Could you check a few things on this model? Use its own coordinates, in mm. Coordinates: 2 decimals unless noted, no trailing zeros. Loops run counter-clockwise (first coordinate to the right, second up) from the corner with the lowest first, then second, coordinate; pieces in that order, holes last. Notation, with made-up numbers: M -34.75,43.25 L -5.75,43.25 A16 ccw -5.75,65.25 Z; hole C -12.5,-18 d5. An arc over 180 degrees is marked long. Use one line per item in the form item = value. Start each with the question number.
Autodesk Inventor part; units mm, degrees
ref_plane "YZ Plane" through (0, 0, 0) normal (1, 0, 0) x (0, 1, 0)
ref_plane "XZ Plane" through (0, 0, 0) normal (0, 1, 0) x (-1, 0, 0)
ref_plane "XY Plane" through (0, 0, 0) normal (0, 0, 1) x (1, 0, 0)
sketch "Sketch1" plane through (0, 0, 0) normal (0, 1, 0) x (-1, 0, 0)
  line L0 (-100.9651, 48.6333) -> (-100.9651, -1.3667)
  line L1 (79.933, 58.6333) -> (-90.9651, 58.6333)
  line L2 (145.3335, 17.5604) -> (88.3289, 56.0635)
  line L3 (-100.9651, -1.3667) -> (-100.9651, -51.3667)
  circle A0 centre (115.0349, 25.6333) radius 1.6
  circle A1 centre (115.0349, -28.3667) radius 1.6
  circle A2 centre (142.5349, 7.3833) radius 1.6
  circle A3 centre (142.5349, -10.1167) radius 1.6
  circle A4 centre (-94.3651, -9.7667) radius 1.6
  circle A5 centre (-94.3651, 7.0333) radius 1.6
  line L4 (147.5349, -16.1504) -> (147.5349, 13.417)
  arc A6 (-100.9651, -51.3667) -> (-90.9651, -61.3667) centre (-90.9651, -51.3667) ccw
  arc A7 (-90.9651, 58.6333) -> (-100.9651, 48.6333) centre (-90.9651, 48.6333) ccw
  arc A8 (88.3289, 56.0635) -> (79.933, 58.6333) centre (79.933, 43.6333) ccw
  arc A9 (79.933, -61.3667) -> (88.3289, -58.7969) centre (79.933, -46.3667) ccw
  arc A10 (147.5349, 13.417) -> (145.3335, 17.5604) centre (142.5349, 13.417) ccw
  arc A11 (145.3335, -20.2938) -> (147.5349, -16.1504) centre (142.5349, -16.1504) ccw
  line L5 (-90.9651, -61.3667) -> (79.933, -61.3667)
  line L6 (88.3289, -58.7969) -> (145.3335, -20.2938)
  line L7 (-90.9651, -1.3667) -> (-90.9651, 16.6333)
  line L8 (-89.9651, 17.6333) -> (-73.9651, 17.6333)
  arc A12 (-71.9651, 15.6333) -> (-73.9651, 17.6333) centre (-73.9651, 15.6333) ccw
  arc A13 (-89.9651, 17.6333) -> (-90.9651, 16.6333) centre (-89.9651, 16.6333) ccw
  line L9 (-71.9651, 15.6333) -> (-71.9651, -13.3667)
  line L10 (-83.9651, -20.3667) -> (-89.9651, -20.3667)
  arc A14 (-90.9651, -19.3667) -> (-89.9651, -20.3667) centre (-89.9651, -19.3667) ccw
  line L11 (-90.9651, -19.3667) -> (-90.9651, -1.3667)
  line L12 (16.0349, -17.3667) -> (16.0349, -43.3667)
  arc A15 (14.0349, -45.3667) -> (16.0349, -43.3667) centre (14.0349, -43.3667) ccw
  line L13 (14.0349, -15.3667) -> (-69.9651, -15.3667)
  arc A16 (16.0349, -17.3667) -> (14.0349, -15.3667) centre (14.0349, -17.3667) ccw
  arc A17 (-71.9651, -13.3667) -> (-69.9651, -15.3667) centre (-69.9651, -13.3667) ccw
  line L14 (14.0349, -45.3667) -> (-79.9651, -45.3667)
  arc A18 (-81.9651, -43.3667) -> (-79.9651, -45.3667) centre (-79.9651, -43.3667) ccw
  line L15 (-81.9651, -43.3667) -> (-81.9651, -22.3667)
  arc A19 (-81.9651, -22.3667) -> (-83.9651, -20.3667) centre (-83.9651, -22.3667) ccw
  line L16 (-54.6151, -49.4667) -> (-64.3151, -49.4667)
  line L17 (-64.3151, -49.4667) -> (-64.3151, -52.2667)
  line L18 (-59.4651, -52.2667) -> (-54.6151, -52.2667)
  line L19 (-54.6151, -52.2667) -> (-54.6151, -49.4667)
  line L20 (-59.4651, -52.2667) -> (-64.3151, -52.2667)
  line L21 (-79.6151, -49.4667) -> (-89.3151, -49.4667)
  line L22 (-89.3151, -49.4667) -> (-89.3151, -52.2667)
  line L23 (-84.4651, -52.2667) -> (-79.6151, -52.2667)
  line L24 (-79.6151, -52.2667) -> (-79.6151, -49.4667)
  line L25 (-84.4651, -52.2667) -> (-89.3151, -52.2667)
  line L26 (-54.6151, 46.7333) -> (-64.3151, 46.7333)
  line L27 (-64.3151, 46.7333) -> (-64.3151, 49.5333)
  line L28 (-59.4651, 49.5333) -> (-54.6151, 49.5333)
  line L29 (-54.6151, 49.5333) -> (-54.6151, 46.7333)
  line L30 (-59.4651, 49.5333) -> (-64.3151, 49.5333)
  line L31 (-79.6151, 46.7333) -> (-89.3151, 46.7333)
  line L32 (-89.3151, 46.7333) -> (-89.3151, 49.5333)
  line L33 (-84.4651, 49.5333) -> (-79.6151, 49.5333)
  line L34 (-79.6151, 49.5333) -> (-79.6151, 46.7333)
  line L35 (-84.4651, 49.5333) -> (-89.3151, 49.5333)
  circle A20 centre (-45.4651, -11.3667) radius 1.6
  circle A21 centre (-45.4651, 40.6333) radius 1.6
  circle A22 centre (86.5349, 40.6333) radius 1.6
  circle A23 centre (20.0349, -41.3667) radius 1.6
  circle A24 centre (86.5349, -41.3667) radius 1.6
  line L36 (129.6349, -6.5167) -> (129.6349, -24.2167)
  line L37 (132.4349, -6.5167) -> (132.4349, -24.2167)
  line L38 (129.6349, 3.7833) -> (129.6349, 21.4833)
  line L39 (132.4349, 3.7833) -> (132.4349, 21.4833)
  line L40 (119.3849, -2.7667) -> (94.6849, -2.7667)
  line L41 (94.6849, 0.0333) -> (119.3849, 0.0333)
  line L42 (94.6849, 0.0333) -> (94.6849, -2.7667)
  line L43 (119.3849, 0.0333) -> (119.3849, -2.7667)
  line L44 (129.6349, -6.5167) -> (132.4349, -6.5167)
  line L45 (132.4349, -24.2167) -> (129.6349, -24.2167)
  line L46 (129.6349, 3.7833) -> (132.4349, 3.7833)
  line L47 (129.6349, 21.4833) -> (132.4349, 21.4833)
  line L48 (-90.8151, -58.2667) -> (-66.1151, -58.2667)
  line L49 (-66.1151, -58.2667) -> (-66.1151, -55.4667)
  line L50 (-66.1151, -55.4667) -> (-90.8151, -55.4667)
  line L51 (-90.8151, -55.4667) -> (-90.8151, -58.2667)
  line L52 (-90.8151, 55.5333) -> (-66.1151, 55.5333)
  line L53 (-66.1151, 55.5333) -> (-66.1151, 52.7333)
  line L54 (-66.1151, 52.7333) -> (-90.8151, 52.7333)
  line L55 (-90.8151, 52.7333) -> (-90.8151, 55.5333)
  line L56 (54.1849, 55.5333) -> (78.8849, 55.5333)
  line L57 (78.8849, 55.5333) -> (78.8849, 52.7333)
  line L58 (78.8849, 52.7333) -> (54.1849, 52.7333)
  line L59 (54.1849, 52.7333) -> (54.1849, 55.5333)
  line L60 (54.1849, -58.2667) -> (78.8849, -58.2667)
  line L61 (78.8849, -58.2667) -> (78.8849, -55.4667)
  line L62 (78.8849, -55.4667) -> (54.1849, -55.4667)
  line L63 (54.1849, -55.4667) -> (54.1849, -58.2667)
extrude "Extrusion1" add sketch "Sketch1" along normal blind 3
properties part number "base" material "Polycarbonate, Clear"
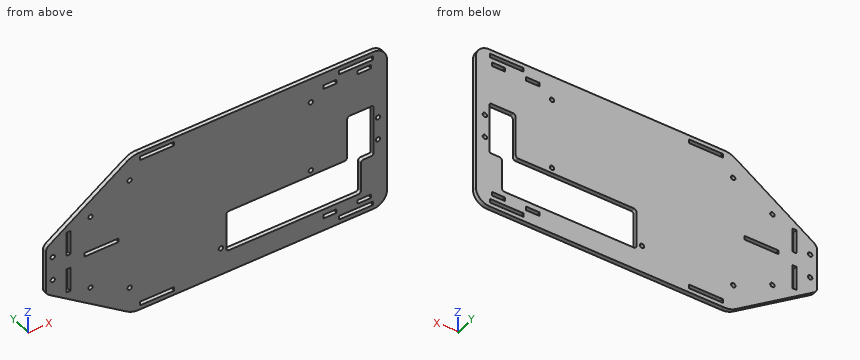
Item 1: I want a section at C-C (y = 2.5). Count the separate pieces of the cut face and the enclosed holes in it, plus the area to 3 significant figures.
Item 2: I'm going to push flat-ended pins straight in: P1, Ø4, axis at x = 1.5, z = 38.5, coming from the -Y side; P2, Ø1.9, axis at x = -142.53, z = 7.38, coming from the +Y side; P3, Ø1.4, axis at y = 1.5, z = -51, coming from the -X side. Where does each tip first touch, or does it pass through?
Item 3: I want a section at D-D (x = -102). Write out the boundary of the cut face in (y, z).
Item 4: I want a section at A-A (x = 39.5). Write out the boundary of the cut face in (y, z), plus the area to 3 significant figures.
Item 5: Please list where these lines run through material, in increasing order: line 1 along Z through (x, y) = (-56.5, 1.45); line 2 along Z through (x, y) = (59, 1); line 3 along Z through (x, y) = (9, 1.9).
Item 6: I want a section at B-B (x = -60.5). Write out the boundary of the cut face in (y, z).
Worked answers:
q1.separate_pieces = 1
q1.enclosed_holes = 23
q1.area = 22,800 mm²
q2.P1 = 0
q2.P2 = through
q2.P3 = -100.91
q3.outline = M 0,-49.56 L 3,-49.56 L 3,-2.77 L 0,-2.77 Z; M 0,0.03 L 3,0.03 L 3,46.83 L 0,46.83 Z
q4.outline = M 0,-61.37 L 3,-61.37 L 3,-45.37 L 0,-45.37 Z; M 0,-15.37 L 3,-15.37 L 3,58.63 L 0,58.63 Z
q4.area = 270 mm²
q5.line_1 = -61.37 to -58.27, -55.47 to 52.73, 55.53 to 58.63
q5.line_2 = -61.37 to -52.27, -49.47 to -45.37, -15.37 to 46.73, 49.53 to 58.63
q5.line_3 = -61.37 to -45.37, -15.37 to 58.63
q6.outline = M 0,-61.37 L 3,-61.37 L 3,-58.27 L 0,-58.27 Z; M 0,-55.47 L 3,-55.47 L 3,52.73 L 0,52.73 Z; M 0,55.53 L 3,55.53 L 3,58.63 L 0,58.63 Z
